The listing builds one solid part. Answer for the finished solid, in the listing's coordinates (mm). A direction names the side the tool comes from. Give positions to 0.01 mm unless a question says otherwise; leave off trailing zeros. Loops run counter-clockwise (first coordinate to the right, second up) from the corner with the lowest first, then second, coordinate; pieces in that order, holes last.
Item 1: A tool of negligible diameter and unlimited length cuts with its end or side. For faces 1 (the face through (-52, 3, -107.136)), 2 (the face through (-52, 3, 95.354)), 3 (the face through (-52, 3, -66.646)), 4 (the face through (38.887, 3, 110)), 5 (the face through (44.887, 3, -6)), from which of +Z, -Z, +X, -X, +Y, -Y can it reach the whole face along a straight path? Write none if from no direction.
Item 2: Each of these flat-tipped pins is pushed along its axis until it touches: pin 1 Ø1.8 at (x, y) = (41.5, 3.5) entering from +Z; pin 2 Ø1.8 at (x, y) = (42, 2) entering from -Z; pin 3 Ø1.8 at (y, z) = (4, -117) entering from +X. Where does it stop, or does it pass through?
Item 3: Consider line 1 along Z through (x, y) = (-50, 2.65); line 2 along X through (y, z) = (2.9, 23); line 3 along Z through (x, y) = (-7, 4.45). Determine where each line is inside the solid, lowest interval first.
Item 4: Section A-A, the plane z = -119 is taken. Give the vertices of the cut face in (x, y), and give its area (3 significant figures).
Item 5: The mould has two halves that part along Z. Classify faces 6 (the face through (-49.103, 3, 34)), 7 (the face through (42, 3, 95.354)), 8 (the face through (-55.103, 3, -87)): pulls with the +Z half, pulls with the -Z half, needs draft (parallel to the pull), parting line crosses it, or undercut.
from build123d import *

# Parameters (mm, degrees)
SKETCH1_W               = 517.884603554
SKETCH1_H               = 307.545036654
BOSS_EXTRUDE1_DEPTH     = 6
CUT_EXTRUDE_THIN1_DEPTH = 302.219360338


with BuildPart() as part:
    # Sketch1 → Boss-Extrude1 (new body)
    with BuildSketch(Plane(origin=(0, 0, 0), x_dir=(1, 0, 0), z_dir=(0, 1, 0))):
        Rectangle(SKETCH1_W, SKETCH1_H)
    extrude(amount=BOSS_EXTRUDE1_DEPTH)

    # Sketch2 → Cut-Extrude-Thin1 (cut, through all)
    with BuildSketch(Plane(origin=(0, 6, 0), x_dir=(1, 0, 0), z_dir=(0, 1, 0))):
        Polygon((38.897086644, -123.820706525), (38.897086644, -95.364474608), (44.897086809, -95.364474608), (44.897086809, -54.854473491), (38.897086644, -54.854473491), (38.897086644, -14.364472375), (44.897086809, -14.364472375), (44.897086809, 26.145528742), (38.897086644, 26.145528742), (38.897086644, 66.635529858), (44.897086809, 66.635529858), (44.897086809, 107.145530974), (38.897086644, 107.145530974), (38.897086644, 135.602227437), (15.137085989, 135.602227437), (15.137085989, 135.600548849), (-25.352915127, 135.600548849), (-25.352915127, 135.602227437), (-49.112915782, 135.602227437), (-49.112915782, 107.145530974), (-55.112946465, 107.145530974), (-55.112946465, 66.635529858), (-49.112915782, 66.635529858), (-49.112915782, 26.145528742), (-55.112946465, 26.145528742), (-55.112946465, -14.364472375), (-49.112915782, -14.364472375), (-49.112915782, -54.854473491), (-55.112946465, -54.854473491), (-55.112946465, -95.364474608), (-49.112915782, -95.364474608), (-49.112915782, -123.820706525), (-25.352915127, -123.820706525), (-25.352915127, -123.819461964), (15.137085989, -123.819461964), (15.137085989, -123.820706525), align=None)
        Polygon((38.887086644, -123.810706525), (38.887086644, -95.354474608), (44.887086809, -95.354474608), (44.887086809, -54.864473491), (38.887086644, -54.864473491), (38.887086644, -14.354472375), (44.887086809, -14.354472375), (44.887086809, 26.135528742), (38.887086644, 26.135528742), (38.887086644, 66.645529858), (44.887086809, 66.645529858), (44.887086809, 107.135530974), (38.887086644, 107.135530974), (38.887086644, 135.592227437), (15.147085989, 135.592227437), (15.147085989, 135.590548849), (-25.362915127, 135.590548849), (-25.362915127, 135.592227437), (-49.102915782, 135.592227437), (-49.102915782, 107.135530974), (-55.102946465, 107.135530974), (-55.102946465, 66.645529858), (-49.102915782, 66.645529858), (-49.102915782, 26.135528742), (-55.102946465, 26.135528742), (-55.102946465, -14.354472375), (-49.102915782, -14.354472375), (-49.102915782, -54.864473491), (-55.102946465, -54.864473491), (-55.102946465, -95.354474608), (-49.102915782, -95.354474608), (-49.102915782, -123.810706525), (-25.362915127, -123.810706525), (-25.362915127, -123.809461964), (15.147085989, -123.809461964), (15.147085989, -123.810706525), align=None, mode=Mode.SUBTRACT)
    extrude(amount=-CUT_EXTRUDE_THIN1_DEPTH, mode=Mode.SUBTRACT)


with BuildPart() as body_2:
    # of the pieces the cut leaves, the one that is kept (cut_extrude_thin1_keep)
    add(part.part.solids().sort_by_distance((15.147085989, 0, 123.809461964))[0])


solid = body_2.part
Worked answers:
1. face 1: -Z, -X, +Y, -Y
1. face 2: +Z, -X, +Y, -Y
1. face 3: -X, +Y, -Y
1. face 4: +Z, +X, +Y, -Y
1. face 5: +Z, -Z, +X, +Y, -Y
2. pin 1: stops at z = 95.35
2. pin 2: stops at z = -107.14
2. pin 3: stops at x = 38.89
3. line 1: z = -107.14 to -66.65, -26.14 to 14.35, 54.86 to 95.35
3. line 2: x = -49.1 to 38.89
3. line 3: z = -135.59 to 123.81
4. outline: (-49.1, 0) - (38.89, 0) - (38.89, 6) - (-49.1, 6) - close
4. area: 528 mm2
5. face 6: undercut
5. face 7: pulls with the +Z half
5. face 8: needs draft
